The listing builds one solid part. Answer for the finished solid, in the listing's coordinates (mm). A direction names the side the tool comes from. Coordinates: 2 decimals unless noted, no trailing zeros. Write each loop counter-clockwise with the first axis right and the second up, starting at its lowest first coordinate (ties: lowest second). Pieces come first, ordered by that corner, then holes.
(1) Given P1, Ø3, axis at x = 20.5, z = 22.5, coming from the -Y side, flat-ended and moving along its own axis, determine where the tip first touches the part or whether it passes through.
(2) For a pull along Y with two mould halves and no side action, classify faces 3 (the flat face through (25, 45.35, 13)), 4 (the cylindrical face through (22.65, 171.75, 12.88)), 5 (the flat face through (25, 203.2, 13)) as +Y half, -Y half, draft (parallel to the pull), parting line (faces both ways), or undercut.
(3) Which of the six approach directions +Z, -Z, +X, -X, +Y, -Y give full straight-line access (tool end or side, diameter ignored) to faces 1 (the flat face through (25, 103, 25.4)), 2 (the flat face through (34.925, 22, 13))?
(4) The part is cut by section C-C on z = 22. Determine the outline of the cut face in (x, y) (3 decimals), plus the area to 3 significant figures.
(5) The part is cut by section B-B on x = 25.4. Determine the outline of the cut face in (y, z), plus the area to 3 significant figures.
(6) The part is cut by section D-D on y = 30. Determine the outline of the cut face in (x, z) (3 decimals), plus the area to 3 significant figures.
(7) Straight lines are drawn through the part: line 1 (Y direction, x = 25.4, z = 19.75); line 2 (X direction, y = 120.5, z = 23); line 3 (X direction, y = 25.5, z = 15.25) (3 decimals). For each, find the intervals that lie inside material, in ascending order.
(8) The part is cut by section A-A on y = 120.65. Determine the outline of the cut face in (x, z).
from build123d import *

# Parameters (mm, degrees)
SKETCH1_W               = 50.8
SKETCH1_H               = 203.2
BOSS_EXTRUDE1_DEPTH     = 25.4
SKETCH2_R               = 12.7
CUT_EXTRUDE1_DEPTH      = 1
CUT_EXTRUDE1_DEPTH_BACK = 26.4
SKETCH3_R               = 6.35
CUT_EXTRUDE2_DEPTH      = 26.4
SKETCH4_W               = 19.05
SKETCH4_H               = 45.349823228
CUT_EXTRUDE3_DEPTH      = 26.4


with BuildPart() as part:
    # Sketch1 → Boss-Extrude1 (new body)
    with BuildSketch(Plane.XY):
        with Locations((25.4, 101.6)):
            Rectangle(SKETCH1_W, SKETCH1_H)
    extrude(amount=BOSS_EXTRUDE1_DEPTH)

    # Sketch2 → Cut-Extrude1 (cut, two sides)
    with BuildSketch(Plane.XY.offset(25.4)) as cut_extrude1_sk:
        with Locations((25.4, 184.15)):
            Circle(SKETCH2_R)
        with Locations((25.4, 120.65)):
            Circle(SKETCH2_R)
    extrude(amount=CUT_EXTRUDE1_DEPTH, mode=Mode.SUBTRACT)
    extrude(cut_extrude1_sk.sketch, amount=-CUT_EXTRUDE1_DEPTH_BACK, mode=Mode.SUBTRACT)

    # Sketch3 → Cut-Extrude2 (cut, through all)
    with BuildSketch(Plane.XY.offset(25.4)):
        with Locations((25.4, 25.4)):
            Circle(SKETCH3_R)
    extrude(amount=-CUT_EXTRUDE2_DEPTH, mode=Mode.SUBTRACT)

    # Sketch4 → Cut-Extrude3 (cut, through all)
    with BuildSketch(Plane.XY.offset(25.4)):
        with Locations((25.4, 22.674911614)):
            Rectangle(SKETCH4_W, SKETCH4_H)
    extrude(amount=-CUT_EXTRUDE3_DEPTH, mode=Mode.SUBTRACT)


solid = part.part
Model answer:
1. P1: stops at y = 45.35
2. face 3: -Y half
2. face 4: undercut
2. face 5: +Y half
3. face 1: +Z, +X, -X, +Y, -Y
3. face 2: +Z, -Z, -Y
4. outline: (0, 0) - (15.875, 0) - (15.875, 45.35) - (34.925, 45.35) - (34.925, 0) - (50.8, 0) - (50.8, 203.2) - (0, 203.2) - close; hole circle Ø25.4 at (25.4, 120.65); hole circle Ø25.4 at (25.4, 184.15)
4. area: 8,450 mm2
5. outline: (45.35, 0) - (107.95, 0) - (107.95, 25.4) - (45.35, 25.4) - close; (133.35, 0) - (171.45, 0) - (171.45, 25.4) - (133.35, 25.4) - close; (196.85, 0) - (203.2, 0) - (203.2, 25.4) - (196.85, 25.4) - close
5. area: 2,720 mm2
6. outline: (0, 0) - (15.875, 0) - (15.875, 25.4) - (0, 25.4) - close; (34.925, 0) - (50.8, 0) - (50.8, 25.4) - (34.925, 25.4) - close
6. area: 806 mm2
7. line 1: y = 45.35 to 107.95, 133.35 to 171.45, 196.85 to 203.2
7. line 2: x = 0 to 12.7, 38.1 to 50.8
7. line 3: x = 0 to 15.875, 34.925 to 50.8
8. outline: (0, 0) - (12.7, 0) - (12.7, 25.4) - (0, 25.4) - close; (38.1, 0) - (50.8, 0) - (50.8, 25.4) - (38.1, 25.4) - close
